from build123d import *

# Parameters (mm, degrees)
SKETCH1_R           = 71
BOSS_EXTRUDE1_DEPTH = 1.5
SKETCH2_R           = 2.2
CUT_EXTRUDE1_DEPTH  = 14.5
SKETCH3_R           = 3.6
SKETCH3_R_2         = 1.6
BOSS_EXTRUDE2_DEPTH = 2
SKETCH4_W           = 10
SKETCH4_H           = 2.2
SKETCH4_H_2         = 0.995039414
SKETCH4_H_3         = 0.995528857
BOSS_EXTRUDE3_DEPTH = 2


with BuildPart() as part:
    # Sketch1 → Boss-Extrude1 (new body)
    with BuildSketch(Plane(origin=(0, 0, 0), x_dir=(1, 0, 0), z_dir=(0, 1, 0))):
        with Locations(Location((0, 0, 0), (0, 0, 270))):
            Circle(SKETCH1_R)
    extrude(amount=BOSS_EXTRUDE1_DEPTH)

    # Sketch2 → Cut-Extrude1 (cut)
    with BuildSketch(Plane(origin=(0, 1.5, 0), x_dir=(1, 0, 0), z_dir=(0, 1, 0))):
        with Locations(Location((0, 0, 0), (0, 0, 270))):
            Circle(SKETCH2_R)
    extrude(amount=-CUT_EXTRUDE1_DEPTH, mode=Mode.SUBTRACT)

    # Sketch3 → Boss-Extrude2 (add)
    # profile 1 of 3: a face of its own
    with BuildSketch(Plane(origin=(0, 1.5, 0), x_dir=(1, 0, 0), z_dir=(0, 1, 0))):
        with Locations(Location((-8.5, 2, 0), (0, 0, 270))):
            Circle(SKETCH3_R)
        with Locations(Location((-8.5, 2, 0), (0, 0, 270))):
            Circle(SKETCH3_R_2, mode=Mode.SUBTRACT)
    # profile 2 of 3: a face of its own
    with BuildSketch(Plane(origin=(0, 1.5, 0), x_dir=(1, 0, 0), z_dir=(0, 1, 0))):
        with Locations(Location((8.5, 2, 0), (0, 0, 270))):
            Circle(SKETCH3_R)
        with Locations(Location((8.5, 2, 0), (0, 0, 270))):
            Circle(SKETCH3_R_2, mode=Mode.SUBTRACT)
    # profile 3 of 3: a face of its own
    with BuildSketch(Plane(origin=(0, 1.5, 0), x_dir=(1, 0, 0), z_dir=(0, 1, 0))):
        with Locations(Location((0, -17.24, 0), (0, 0, 270))):
            Circle(SKETCH3_R)
        with Locations(Location((0, -17.24, 0), (0, 0, 270))):
            Circle(SKETCH3_R_2, mode=Mode.SUBTRACT)
    extrude(amount=BOSS_EXTRUDE2_DEPTH)

    # Sketch4 → Boss-Extrude3 (add)
    with BuildSketch(Plane(origin=(0, 1.5, 0), x_dir=(1, 0, 0), z_dir=(0, 1, 0))):
        with Locations((-17.3, -7.5)):
            Rectangle(SKETCH4_W, SKETCH4_H)
        with Locations((-17.3, -11.697519707)):
            Rectangle(SKETCH4_W, SKETCH4_H_2)
        with Locations((-17.3, -3.302235572)):
            Rectangle(SKETCH4_W, SKETCH4_H_3)
        with Locations((-17.3, 0.302235572)):
            Rectangle(SKETCH4_W, SKETCH4_H_3)
        with Locations((-17.3, -15.302480293)):
            Rectangle(SKETCH4_W, SKETCH4_H_2)
        with Locations((17.3, -15.302480293)):
            Rectangle(SKETCH4_W, SKETCH4_H_2)
        with Locations((17.3, -11.697519707)):
            Rectangle(SKETCH4_W, SKETCH4_H_2)
        with Locations((17.3, -7.5)):
            Rectangle(SKETCH4_W, SKETCH4_H)
        with Locations((17.3, -3.302235572)):
            Rectangle(SKETCH4_W, SKETCH4_H_3)
        with Locations((17.3, 0.302235572)):
            Rectangle(SKETCH4_W, SKETCH4_H_3)
    extrude(amount=BOSS_EXTRUDE3_DEPTH)


solid = part.part
Can you work these out from the model? Positions are in its coordinate system, mm. A direction names the side the tool comes from. Give positions to 0.01 mm unless a question says otherwise; leave off trailing zeros. Order: outer loops, then holes, each group sorted by start corner. A loop starts at its lowest first (then second) coordinate and runs counter-clockwise, first axis right, second up. Notation, with made-up numbers: M 88.25,55 L 118.25,55 A15 ccw 118.25,75 Z; hole C -34,58.25 d2. An arc over 180 degrees is marked long. One line per question, with ' | ' between items.
Item 1: Please list where these lines run through material, in increasing order: L1, parallel to X at y = 2, z = -2; L2, parallel to Y at x = 43.5, z = -32; L3, parallel to X at y = 0.55, z = 0.
Answer block:
L1: x = -12.1 to -10.1, -6.9 to -4.9, 4.9 to 6.9, 10.1 to 12.1 | L2: y = 0 to 1.5 | L3: x = -71 to -2.2, 2.2 to 71
Item 2: For faces 1 (the face through (0.158, 2.486, 13.643)), 2 (the face through (-62.99, 0.74, 32.76)), which set-ups out of +Z, -Z, +X, -X, +Y, -Y let a thin tool reach every point of the face, with its end or its side?
Answer block:
face 1: +Y | face 2: +Y, -Y
Item 3: I'm going to push flat-ended pins straight in: pin 1 Ø0.6 at (x, y) = (15.5, 2.5) entering from +Z; pin 2 Ø1.1 at (y, z) = (2.5, 15.5) entering from +X; pin 3 Ø2 at (y, z) = (2, 7.5) entering from -X. Where does each tip first touch, or does it pass through?
Answer block:
pin 1: stops at z = 15.8 | pin 2: stops at x = 22.3 | pin 3: stops at x = -70.69
Item 4: We'd pull the mould along Z, two halves only. Please class faces 3 (the face through (0, 1.5, 17)), 4 (the face through (-8, 1.5, -2)), 5 (the face through (4.986, 2.486, -2.78)), 6 (the face through (-15, 0, -1)): released by +Z, released by -Z, zero draft, split by the parting line, or undercut.
Answer block:
face 3: undercut | face 4: undercut | face 5: split by the parting line | face 6: zero draft
Item 5: Suppose I cut it at A-A, the plane y = 2.25. Give the number of separate pieces and of enclosed holes in the cut face, then the cut area to 3 significant figures.
Answer block:
separate pieces: 13 | enclosed holes: 3 | area: 222 mm2
Item 6: Suppose I cut it at B-B, the plane z = -22.5. Write out the boundary of the cut face in (x, y).
Answer block:
outline: M -67.34,0 L 67.34,0 L 67.34,1.5 L -67.34,1.5 Z
Item 7: Suppose I cut it at C-C, the plane x = -40.5. Write out the boundary of the cut face in (y, z).
Answer block:
outline: M 0,-58.32 L 1.5,-58.32 L 1.5,58.32 L 0,58.32 Z
